from build123d import *

# Parameters (mm, degrees)
F2_DEPTH = 10


with BuildPart() as f2:
    # F1 (on Top) → F2 (new body)
    with BuildSketch(Plane.XY):
        Polygon((-7, 7.2), (0, 7.2), (0, 9.6), (-9.4, 9.6), (-9.4, 2.4), (-50.15, 2.4), (-50.15, -21.5), (-47.75, -21.5), (-43.25, -17.5), (-43.25, -15.5), (-47.75, -14.5), (-47.75, 0), (-7, 0), align=None)
    extrude(amount=F2_DEPTH)

    # F3: F2 across plane


with BuildPart() as f2_1:
    add(f2.part)
    add(f2.part.mirror(Plane.YZ))


solid = f2_1.part
Can you work these out from the model? Positions are in its coordinate system, mm. A direction names the side the tool comes from. Give positions to 0.01 mm unless a question says otherwise; leave off trailing zeros. Loops run counter-clockwise (first coordinate to the right, second up) from the corner with the lowest first, then second, coordinate; pieces in that order, holes last. Notation, with made-up numbers: M -0.5,0 L 47.5,0 A18 ccw 47.5,23 Z; hole C -1.5,87.5 d4. An arc over 180 degrees is marked long. One line per item, written item: value.
1) Imagine slicing it at A-A on y = -8. Write out the boundary of the cut face in (x, z).
Geometry check:
outline: M -50.15,0 L -47.75,0 L -47.75,10 L -50.15,10 Z; M 47.75,0 L 50.15,0 L 50.15,10 L 47.75,10 Z
2) Imagine slicing it at B-B on z = 4.5. Write out the boundary of the cut face in (x, y), and give its area (3 significant figures).
Geometry check:
outline: M -50.15,-21.5 L -47.75,-21.5 L -43.25,-17.5 L -43.25,-15.5 L -47.75,-14.5 L -47.75,0 L -7,0 L -7,7.2 L 7,7.2 L 7,0 L 47.75,0 L 47.75,-14.5 L 43.25,-15.5 L 43.25,-17.5 L 47.75,-21.5 L 50.15,-21.5 L 50.15,2.4 L 9.4,2.4 L 9.4,9.6 L -9.4,9.6 L -9.4,2.4 L -50.15,2.4 Z
area: 419 mm²
3) I'm going to push flat-ended pins straight in: pin 1 (5 mm diameter, centred on x = 32, z = 6, fed in from -Y); pin 2 (5 mm diameter, centred on x = -1.5, z = 6, fed in from -Y); pin 3 (6 mm diameter, centred on y = 7, z = 6.5, fed in from +X). Where does each tip first touch, or does it pass through?
Geometry check:
pin 1: stops at y = 0
pin 2: stops at y = 7.2
pin 3: stops at x = 9.4
4) Imagine slicing it at D-D on x = 0.5. Write out the boundary of the cut face in (y, z), and give its area (3 significant figures).
Geometry check:
outline: M 7.2,0 L 9.6,0 L 9.6,10 L 7.2,10 Z
area: 24.0 mm²
5) Imagine slicing it at C-C on y = 1. Write out the boundary of the cut face in (x, z).
Geometry check:
outline: M -50.15,0 L -7,0 L -7,10 L -50.15,10 Z; M 7,0 L 50.15,0 L 50.15,10 L 7,10 Z
6) Thinking about a two-plate mould opening in Y: for faces 6 (the face through (-45.5, -19.5, 4.9)), 7 (the face through (-47.75, -7, 5)), 8 (the face through (8, 1, 0)), which applies, +Y half, -Y half, draft (parallel to the pull), parting line (faces both ways), or undercut?
Geometry check:
face 6: -Y half
face 7: undercut
face 8: draft
7) Please list where these lines run through material, in increasing order: line 1 (X direction, y = 3, z = 1.75); line 2 (X direction, y = -13, z = 6.5); line 3 (Y direction, x = 39.5, z = 3.5).
Geometry check:
line 1: x = -9.4 to -7, 7 to 9.4
line 2: x = -50.15 to -47.75, 47.75 to 50.15
line 3: y = 0 to 2.4
8) On a 3-axis mill with a long thin cutter (end or side, diameter ignored), from which of +Z, -Z, +X, -X, +Y, -Y can I reach the whole of each face in a straight line? I mean faces 1 (the face through (0, 7.2, 5)), 2 (the face through (9.4, 6, 5)), 3 (the face through (-9.4, 6, 5)), 4 (the face through (-50.15, -9, 5)), 5 (the face through (47.75, -7, 5)). Say none if no direction works.
Geometry check:
face 1: +Z, -Z, -Y
face 2: +Z, -Z, +X, +Y
face 3: +Z, -Z, -X, +Y
face 4: +Z, -Z, -X, +Y, -Y
face 5: +Z, -Z
